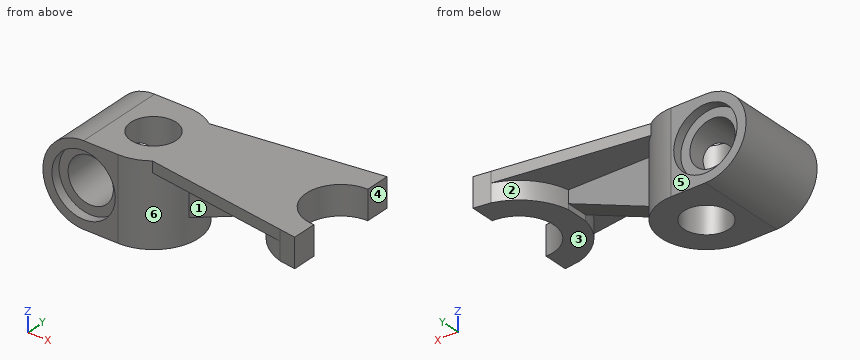
from build123d import *

# Parameters (mm, degrees)
SKETCH1_R           = 12.5
BOSS_EXTRUDE1_DEPTH = 45
BOSS_EXTRUDE2_DEPTH = 50
SKETCH4_R           = 17.5
CUT_EXTRUDE1_DEPTH  = 5
CUT_EXTRUDE2_START  = -5
SKETCH5_R           = 17.5
CUT_EXTRUDE2_DEPTH  = 5
SKETCH6_R           = 12.5
CUT_EXTRUDE3_DEPTH  = 96
BOSS_EXTRUDE3_DEPTH = 16
BOSS_EXTRUDE4_START = -6
BOSS_EXTRUDE4_DEPTH = 6
BOSS_EXTRUDE5_DEPTH = 26
CUT_EXTRUDE6_DEPTH  = 27
CUT_EXTRUDE13_DEPTH = 45
CUT_EXTRUDE14_DEPTH = 45


with BuildPart() as part:
    # Sketch1 → Boss-Extrude1 (new body)
    with BuildSketch(Plane.XY):
        with BuildLine():
            Line((-16.9285558, 31.718520583), (-35.9285558, 31.718520583))
            Line((-35.9285558, 31.718520583), (-35.9285558, -18.281479417))
            Line((-35.9285558, -18.281479417), (-16.9285558, -18.281479417))
            ThreePointArc((-16.9285558, -18.281479417), (8.0714442, 6.718520583), (-16.9285558, 31.718520583))
        make_face()
        with Locations(Location((-16.9285558, 6.718520583, 0), (0, 0, 180))):
            Circle(SKETCH1_R, mode=Mode.SUBTRACT)
    extrude(amount=BOSS_EXTRUDE1_DEPTH)

    # Sketch2 → Boss-Extrude2 (add)
    with BuildSketch(Plane(origin=(0, 31.718520583, 0), x_dir=(1, 0, 0), z_dir=(0, 1, 0))):
        with BuildLine():
            Line((-35.9285558, 0), (-35.9285558, -45))
            ThreePointArc((-35.9285558, -45), (-58.4285558, -22.5), (-35.9285558, 0))
        make_face()
    extrude(amount=-BOSS_EXTRUDE2_DEPTH)

    # Sketch4 → Cut-Extrude1 (cut)
    with BuildSketch(Plane(origin=(0, 31.718520583, 0), x_dir=(1, 0, 0), z_dir=(0, 1, 0))):
        with Locations(Location((-35.9285558, -22.5, 0), (0, 0, 270))):
            Circle(SKETCH4_R)
    extrude(amount=-CUT_EXTRUDE1_DEPTH, mode=Mode.SUBTRACT)

    # Sketch5 → Cut-Extrude2 (cut)
    with BuildSketch(Plane.XZ.offset(18.281479417).offset(CUT_EXTRUDE2_START)):
        with Locations(Location((-35.9285558, 22.5, 0), (0, 0, 90))):
            Circle(SKETCH5_R)
    extrude(amount=CUT_EXTRUDE2_DEPTH, mode=Mode.SUBTRACT)

    # Sketch6 → Cut-Extrude3 (cut)
    with BuildSketch(Plane.XZ.offset(13.281479417)):
        with Locations(Location((-35.9285558, 22.5, 0), (0, 0, 270))):
            Circle(SKETCH6_R)
    extrude(amount=-CUT_EXTRUDE3_DEPTH, mode=Mode.SUBTRACT)



with BuildPart() as body_2:
    # Sketch7 → Boss-Extrude3 (new body)
    with BuildSketch(Plane.XY.offset(45)):
        with BuildLine():
            Line((86.5714442, 39.218520583), (86.5714442, 25.718520583))
            ThreePointArc((86.5714442, 25.718520583), (67.5714442, 6.718520583), (86.5714442, -12.281479417))
            Line((86.5714442, -12.281479417), (86.5714442, -25.781479417))
            ThreePointArc((86.5714442, -25.781479417), (54.0714442, 6.718520583), (86.5714442, 39.218520583))
        make_face()
    extrude(amount=-BOSS_EXTRUDE3_DEPTH)


with BuildPart() as part_1:
    add(part.part)

    add(body_2.part)  # Boss-Extrude4 merges body 2
    # Sketch8 → Boss-Extrude4 (add)
    with BuildSketch(Plane.XY.offset(45).offset(BOSS_EXTRUDE4_START)):
        with BuildLine():
            Line((77.570223695, 37.947161755), (-1.9285558, 26.718520583))
            ThreePointArc((-1.9285558, 26.718520583), (8.0714442, 6.718520583), (-1.9285558, -13.281479417))
            Line((-1.9285558, -13.281479417), (77.570223695, -24.510120588))
            ThreePointArc((77.570223695, -24.510120588), (54.0714442, 6.718520583), (77.570223695, 37.947161755))
        make_face()
    extrude(amount=BOSS_EXTRUDE4_DEPTH)

    # Sketch11 → Boss-Extrude5 (add)
    with BuildSketch(Plane(origin=(0, 0, 39), x_dir=(-1, 0, 0), z_dir=(0, 0, -1))):
        with BuildLine():
            Line((-7.340766399, 12.718520583), (-54.630091692, 12.718520583))
            ThreePointArc((-54.630091692, 12.718520583), (-54.0714442, 6.718520583), (-54.630091692, 0.718520583))
            Line((-54.630091692, 0.718520583), (-7.340766399, 0.718520583))
            ThreePointArc((-7.340766399, 0.718520583), (-8.0714442, 6.718520583), (-7.340766399, 12.718520583))
        make_face()
    extrude(amount=BOSS_EXTRUDE5_DEPTH)

    # Sketch12 → Cut-Extrude6 (cut)
    with BuildSketch(Plane.XZ.offset(-0.718520583)):
        Polygon((54.630091692, 32), (7.340766399, 13), (54.630091692, 13), align=None)
    extrude(amount=-CUT_EXTRUDE6_DEPTH, mode=Mode.SUBTRACT)

    # Sketch22 → Cut-Extrude13 (cut)
    with BuildSketch(Plane.XY.offset(45)):
        Polygon((86.5714442, 39.218520583), (77.570223695, 37.947161755), (65.199967012, 56.955266835), (110.383312753, 52.793642885), align=None)
    extrude(amount=-CUT_EXTRUDE13_DEPTH, mode=Mode.SUBTRACT)

    # Sketch23 → Cut-Extrude14 (cut)
    with BuildSketch(Plane.XY.offset(45)):
        Polygon((86.5714442, -25.781479417), (77.570223695, -24.510120588), (41.145903609, -43.152647533), (115.929494314, -52.929136625), align=None)
    extrude(amount=-CUT_EXTRUDE14_DEPTH, mode=Mode.SUBTRACT)


solid = part_1.part
For this review, take the finished solid that the model builds, in its own axes (mm). Face numbers are marked on the shaded views. A direction names the side the tool comes from. Coordinates: 2 decimals unless noted, no trailing zeros. Loops run counter-clockwise (first coordinate to the right, second up) from the corner with the lowest first, then second, coordinate; pieces in that order, holes last. Notation, with made-up numbers: (19.25, -0.75) -> (50.25, -0.75) arc R23 ccw to (50.25, 22.25) -> close; hole circle Ø7 at (-37.5, 26). An arc over 180 degrees is marked (long way). Write each question's results on one line, items separated by ' | '.
Q1. To check wall thickness, follow line 1 along Z through (x, y) = (-36.5, 15); line 2 along Z through (x, y) = (64.5, 21); line 3 along Y through (x, z) = (-13.5, 11). State the ranges of each line that lie inside material, in increasing order. Write a range as [from, to].
Taken from the geometry:
line 1: [0.01, 10.01], [34.99, 44.99] | line 2: [29, 45] | line 3: [-18.05, -5.3], [18.74, 31.48]
Q2. Mouldability with a two-part tool opening along X and no side actions: class the marked faces 4, 5 and 6 as +X half, -X half, draft (parallel to the pull), parting line (faces both ways), or undercut.
Taken from the geometry:
face 4: +X half | face 5: draft | face 6: undercut
Q3. Add section A-A, the plane z = 22. State the section outline as (x, y) points.
Taken from the geometry:
outline: (-58.42, -18.28) -> (-53.42, -18.28) -> (-53.42, -13.28) -> (-48.42, -13.28) -> (-48.42, 26.72) -> (-53.42, 26.72) -> (-53.42, 31.72) -> (-58.42, 31.72) -> close; (-23.44, -13.28) -> (-18.44, -13.28) -> (-18.44, -18.28) -> (-16.93, -18.28) arc R25 ccw to (7.34, 0.72) -> (29.74, 0.72) -> (29.74, 12.72) -> (7.34, 12.72) arc R25 ccw to (-16.93, 31.72) -> (-18.44, 31.72) -> (-18.44, 26.72) -> (-23.44, 26.72) -> (-23.44, 17.39) arc R12.5 cw (long way) to (-23.44, -3.95) -> close
Q4. For pin 1 Ø1.5 at (y, z) = (8.5, 31) entering from -X; pin 2 Ø10 at (y, z) = (20, 22) entering from +X; pin 3 Ø1.5 at (y, z) = (-6, 27.5) entering from -X; pin 4 Ø20 at (x, y) = (-16.93, 6.72) entering from -Z, all flat-tipped, find the tip position at first contact; note any pin that passes through.
Taken from the geometry:
pin 1: x = -57.05 | pin 2: x = 6.66 | pin 3: x = -58.02 | pin 4: through
Q5. Add section B-B, the plane x = 72. State the section outline as (y, z) points.
Taken from the geometry:
outline: (-23.72, 39) -> (-22.33, 39) -> (-22.33, 29) -> (-5.47, 29) -> (-5.47, 45) -> (-23.72, 45) -> close; (18.91, 29) -> (35.77, 29) -> (35.77, 39) -> (37.16, 39) -> (37.16, 45) -> (18.91, 45) -> close
Q6. Add section D-D, the plane x = 19. State the section outline as (y, z) points.
Taken from the geometry:
outline: (-16.24, 39) -> (0.72, 39) -> (0.72, 17.68) -> (12.72, 17.68) -> (12.72, 39) -> (29.67, 39) -> (29.67, 45) -> (-16.24, 45) -> close
Q7. Machinability: for the marked faces 1, 2 and 3, which of the approach directions +Z, -Z, +X, -X, +Y, -Y give a long, thin tool a straight path to every point of the face, cutting with its end or side? Answer none if there is none.
Taken from the geometry:
face 1: -Z, -Y | face 2: -Z, +Y | face 3: -Z, +X, +Y, -Y
Q8. Add section C-C, the plane y = 16. State the section outline as (x, z) points.
Taken from the geometry:
outline: (-35.93, 0) -> (-25.3, 0) -> (-25.3, 15.92) arc R12.5 cw (long way) to (-25.3, 29.08) -> (-25.3, 45) -> (-35.93, 45) arc R22.5 ccw to start; (-8.56, 0) -> (6.28, 0) -> (6.28, 39) -> (55.42, 39) -> (55.42, 29) -> (69.99, 29) -> (69.99, 45) -> (-8.56, 45) -> close
